```python
from build123d import *

# Parameters (mm, degrees)
MODEL_R            = 0.8
MODEL_R_2          = 1.59995
MODEL_W            = 1.6
MODEL_H            = 1.6
BOSS_EXTRU_1_DEPTH = 1.6


with BuildPart() as part:
    # Model → Boss.-Extru.1 (new body)
    with BuildSketch(Plane.XY):
        Polygon((0, 3.2), (0, 39.9), (3.4, 43.3), (3.4, 47.8), (-0.1, 51.3), (-0.1, 59.1), (4.1, 63.3), (96.2, 63.3), (100.3, 59.2), (100.3, 3.2), (97.1, 0), (3.2, 0), align=None)
        with Locations((5.3, 7.6)):
            Circle(MODEL_R, mode=Mode.SUBTRACT)
        with Locations((7.84, 7.6)):
            Circle(MODEL_R, mode=Mode.SUBTRACT)
        with Locations((10.38, 7.6)):
            Circle(MODEL_R, mode=Mode.SUBTRACT)
        with Locations((12.92, 7.6)):
            Circle(MODEL_R, mode=Mode.SUBTRACT)
        with Locations((15.46, 7.6)):
            Circle(MODEL_R, mode=Mode.SUBTRACT)
        with Locations((18, 7.6)):
            Circle(MODEL_R, mode=Mode.SUBTRACT)
        with Locations((20.54, 7.6)):
            Circle(MODEL_R, mode=Mode.SUBTRACT)
        with Locations((23.08, 7.6)):
            Circle(MODEL_R, mode=Mode.SUBTRACT)
        with Locations((27.14, 7.6)):
            Circle(MODEL_R, mode=Mode.SUBTRACT)
        with Locations((29.68, 7.6)):
            Circle(MODEL_R, mode=Mode.SUBTRACT)
        with Locations((32.22, 7.6)):
            Circle(MODEL_R, mode=Mode.SUBTRACT)
        with Locations((34.76, 7.6)):
            Circle(MODEL_R, mode=Mode.SUBTRACT)
        with Locations((37.3, 7.6)):
            Circle(MODEL_R, mode=Mode.SUBTRACT)
        with Locations((39.84, 7.6)):
            Circle(MODEL_R, mode=Mode.SUBTRACT)
        with Locations((42.38, 7.6)):
            Circle(MODEL_R, mode=Mode.SUBTRACT)
        with Locations((44.92, 7.6)):
            Circle(MODEL_R, mode=Mode.SUBTRACT)
        with Locations((47.46, 7.6)):
            Circle(MODEL_R, mode=Mode.SUBTRACT)
        with Locations((50, 7.6)):
            Circle(MODEL_R, mode=Mode.SUBTRACT)
        with Locations((38.32, 55.86)):
            Circle(MODEL_R, mode=Mode.SUBTRACT)
        with Locations((35.78, 55.86)):
            Circle(MODEL_R, mode=Mode.SUBTRACT)
        with Locations((33.24, 55.86)):
            Circle(MODEL_R, mode=Mode.SUBTRACT)
        with Locations((30.7, 55.86)):
            Circle(MODEL_R, mode=Mode.SUBTRACT)
        with Locations((28.16, 55.86)):
            Circle(MODEL_R, mode=Mode.SUBTRACT)
        with Locations((25.62, 55.86)):
            Circle(MODEL_R, mode=Mode.SUBTRACT)
        with Locations((23.08, 55.86)):
            Circle(MODEL_R, mode=Mode.SUBTRACT)
        with Locations((18, 55.86)):
            Circle(MODEL_R, mode=Mode.SUBTRACT)
        with Locations((15.46, 55.86)):
            Circle(MODEL_R, mode=Mode.SUBTRACT)
        with Locations((12.92, 55.86)):
            Circle(MODEL_R, mode=Mode.SUBTRACT)
        with Locations((10.38, 55.86)):
            Circle(MODEL_R, mode=Mode.SUBTRACT)
        with Locations((7.84, 55.86)):
            Circle(MODEL_R, mode=Mode.SUBTRACT)
        with Locations((5.3, 55.86)):
            Circle(MODEL_R, mode=Mode.SUBTRACT)
        with Locations((20, 51.3)):
            Circle(MODEL_R_2, mode=Mode.SUBTRACT)
        with Locations((65.6, 60.5)):
            Circle(MODEL_R_2, mode=Mode.SUBTRACT)
        with Locations((64.4, 16.6)):
            Circle(MODEL_R_2, mode=Mode.SUBTRACT)
        with Locations((3.4, 23.1)):
            Circle(MODEL_R_2, mode=Mode.SUBTRACT)
        with Locations((7.84, 61)):
            Circle(MODEL_R, mode=Mode.SUBTRACT)
        with Locations((10.38, 61)):
            Circle(MODEL_R, mode=Mode.SUBTRACT)
        with Locations((12.92, 61)):
            Circle(MODEL_R, mode=Mode.SUBTRACT)
        with Locations((15.46, 61)):
            Circle(MODEL_R, mode=Mode.SUBTRACT)
        with Locations((18, 61)):
            Circle(MODEL_R, mode=Mode.SUBTRACT)
        with Locations((47.46, 2.5)):
            Circle(MODEL_R, mode=Mode.SUBTRACT)
        with Locations((44.92, 2.5)):
            Circle(MODEL_R, mode=Mode.SUBTRACT)
        with Locations((42.38, 2.5)):
            Circle(MODEL_R, mode=Mode.SUBTRACT)
        with Locations((39.84, 2.5)):
            Circle(MODEL_R, mode=Mode.SUBTRACT)
        with Locations((37.3, 2.5)):
            Circle(MODEL_R, mode=Mode.SUBTRACT)
        with Locations((34.76, 2.5)):
            Circle(MODEL_R, mode=Mode.SUBTRACT)
        with Locations((32.22, 2.5)):
            Circle(MODEL_R, mode=Mode.SUBTRACT)
        with Locations((20.56, 2.5)):
            Circle(MODEL_R, mode=Mode.SUBTRACT)
        with Locations((18.02, 2.5)):
            Circle(MODEL_R, mode=Mode.SUBTRACT)
        with Locations((15.48, 2.5)):
            Circle(MODEL_R, mode=Mode.SUBTRACT)
        with Locations((12.94, 2.5)):
            Circle(MODEL_R, mode=Mode.SUBTRACT)
        with Locations((10.4, 2.5)):
            Circle(MODEL_R, mode=Mode.SUBTRACT)
        with Locations((7.86, 2.5)):
            Circle(MODEL_R, mode=Mode.SUBTRACT)
        with Locations((5.32, 2.5)):
            Circle(MODEL_R, mode=Mode.SUBTRACT)
        with Locations((25.64, 61)):
            Circle(MODEL_R, mode=Mode.SUBTRACT)
        with Locations((28.18, 61)):
            Circle(MODEL_R, mode=Mode.SUBTRACT)
        with Locations((30.72, 61)):
            Circle(MODEL_R, mode=Mode.SUBTRACT)
        with Locations((33.26, 61)):
            Circle(MODEL_R, mode=Mode.SUBTRACT)
        with Locations((35.8, 61)):
            Circle(MODEL_R, mode=Mode.SUBTRACT)
        with Locations((38.34, 61)):
            Circle(MODEL_R, mode=Mode.SUBTRACT)
        with Locations((40.88, 61)):
            Circle(MODEL_R, mode=Mode.SUBTRACT)
        with Locations((40.86, 55.86)):
            Rectangle(MODEL_W, MODEL_H, mode=Mode.SUBTRACT)
        with Locations((5.3, 61)):
            Rectangle(MODEL_W, MODEL_H, mode=Mode.SUBTRACT)
        with Locations((50, 2.5)):
            Rectangle(MODEL_W, MODEL_H, mode=Mode.SUBTRACT)
        with Locations((23.1, 2.5)):
            Rectangle(MODEL_W, MODEL_H, mode=Mode.SUBTRACT)
        with Locations((23.1, 61)):
            Rectangle(MODEL_W, MODEL_H, mode=Mode.SUBTRACT)
    extrude(amount=BOSS_EXTRU_1_DEPTH)


solid = part.part
```
Could you check a few things on this model? Use its own coordinates, in mm. A direction names the side the tool comes from. Give positions to 0.01 mm unless a question says otherwise; leave off trailing zeros. Loops run counter-clockwise (first coordinate to the right, second up) from the corner with the lowest first, then second, coordinate; pieces in that order, holes last. Notation, with made-up numbers: (87, -5) - (138, -5) arc R8 ccw to (138, 5) - close; hole circle Ø10 at (88, -1). An arc over 180 degrees is marked (long way). Answer in a Markdown table with one row per item. Add a question column.
Q1. For pin 1 (1 mm diameter, centred on x = 28.16, y = 55.86, fed in from -Z), with a flat end and sliding along its axis, tell me the tip position at first contact or that it passes through.
Q2. We'd pull the mould along X, two halves only. Please class faces 3 (the face through (64.05, 15.04, 0.79)), 4 (the face through (98.2, 61.3, 0.8)), 5 (the face through (1.7, 49.5, 0.8)), 6 (the face through (51, 32, 1.6)): +X half, -X half, draft (parallel to the pull), parting line (faces both ways), or undercut.
Q3. Which directions (+Z, -Z, +X, -X, +Y, -Y) give clear straight access to the entire face, cutting with the end or side of a thin tool? Please do faces 1 (the face through (1.7, 41.6, 0.8)), 2 (the face through (1.6, 1.6, 0.8)).
Q4. If we section it at A-A (y = 45): List the corners of the cut face in (x, z) for me, plus the area to 3 significant figures.
Q5. Please list where these lines run through material, in increasing order: L1, parallel to Y at x = 10.38, z = 0.5; L2, parallel to Y at x = 33.24, z = 0.55; L3, parallel to Y at x = 47.46, z = 0.45. Write a range as from..to.
Q6. If we section it at B-B (z = 0.4): State how many separate pieces and enclosed holes the cut face has, plus the area to 3 significant figures.
The answers:
| question | item | result |
|---|---|---|
| 1 | pin 1 | passes through |
| 2 | face 3 | undercut |
| 2 | face 4 | +X half |
| 2 | face 5 | -X half |
| 2 | face 6 | draft |
| 3 | face 1 | +Z, -Z, -X |
| 3 | face 2 | +Z, -Z, -X, -Y |
| 4 | outline | (3.4, 0) - (100.3, 0) - (100.3, 1.6) - (3.4, 1.6) - close |
| 4 | area | 155 mm^2 |
| 5 | L1 | y = 0..1.7, 3.3..6.8, 8.4..55.06, 56.66..60.2, 61.8..63.3 |
| 5 | L2 | y = 0..55.06, 56.66..60.2, 61.8..63.3 |
| 5 | L3 | y = 0..1.7, 3.3..6.8, 8.4..63.3 |
| 6 | separate pieces | 1 |
| 6 | enclosed holes | 66 |
| 6 | area | 6,140 mm^2 |
